Can you work these out from the model? Positions are in its coordinate system, mm. Coordinates: 2 decimals unless noted, no trailing zeros. Order: outer loops, then holes, each group sorted by start corner. A loop starts at its lowest first (then second) coordinate and runs counter-clockwise, first axis right, second up. Notation, with made-up numbers: (-35.5, -5.5) - (-15.5, -5.5) arc R30 cw to (-15.5, 16.5) - close; hole circle Ø6 at (-36.75, 38.5). An arc over 180 degrees is marked (long way). Return JSON: item names as keys, results as strings. Group by question number.
1) Imagine slicing it at B-B (y = 1.8). Give the number of separate pieces and of enclosed holes in the cut face, and give its area (3 significant figures).
2) For pin 1 Ø1.6 at (x, y) = (102, 1.5) entering from -Z; pin 2 Ø3 at (x, z) = (86.96, 38.69) entering from +Y; pin 3 Ø1.5 at (y, z) = (2.5, -19) entering from +X; pin 4 Ø0.6 at (x, y) = (102, 2) entering from +Z, each with a flat end and sliding along its axis, tell me the tip position at first contact or that it passes through.
3) If we mould it in two halves opening along Z, with no side actions, what happens to faces 1 (the face through (-83, 0, 41)), 2 (the face through (-172.517, 2.535, -37.813))? For each: pulls with the +Z half, pulls with the -Z half, needs draft (parallel to the pull), parting line crosses it, or undercut.
4) If I drill on line 1 along Z through (x, y) = (165.5, 4.15); line 2 along Z through (x, y) = (192, 3.5); line 3 along X through (y, z) = (3.85, 127), over which ranges is the centre line in solid material (lowest first)?
5) Imagine slicing it at A-A (z = -63.5). Write out the boundary of the cut face in (x, y), and give its area (3 significant figures).
6) Imagine slicing it at C-C (z = 20.5). Write out the boundary of the cut face in (x, y).
Autodesk Inventor part; units mm, degrees
ref_plane "Work Plane2" through (100.7136, 5, 38.6884) normal (0, 0, 1) x (1, 0, 0)
ref_plane "YZ Plane" through (0, 0, 0) normal (1, 0, 0) x (0, 1, 0)
ref_plane "XZ Plane" through (0, 0, 0) normal (0, 1, 0) x (-1, 0, 0)
sketch "Sketch1" plane through (0, 0, 0) normal (0, 1, 0) x (-1, 0, 0)
  line L0 (277.2864, 213.6884) -> (-214.7136, 213.6884)
  line L1 (-214.7136, -136.3116) -> (277.2864, -136.3116)
  line L2 (277.2864, -136.3116) -> (277.2864, 213.6884)
  line L3 (-214.7136, 159.6884) -> (-102.7136, 159.6884)
  line L4 (-102.7136, 159.6884) -> (-102.7136, -82.3116)
  line L5 (-102.7136, -82.3116) -> (-214.7136, -82.3116)
  line L6 (-214.7136, 213.6884) -> (-214.7136, 159.6884)
  line L7 (-214.7136, -82.3116) -> (-214.7136, -136.3116)
  point P0 (0, 0)
  dimension "d0" = 350
  dimension "d1" = 492
  dimension "d2" = 112
  dimension "d3" = 112
  dimension "d4" = 54
  dimension "d5" = 54
extrude "Extrusion1" add sketch "Sketch1" along normal blind 5
sketch "Sketch2" plane through (0, 5, 0) normal (0, 1, 0) x (1, 0, 0)
  line L0 (214.7136, 136.3116) -> (-277.2864, 136.3116)
  line L1 (-207.2864, 136.3116) -> (-137.2864, 136.3116)
  line L2 (-137.2864, 136.3116) -> (-137.2864, 134.3116)
  line L3 (-137.2864, 134.3116) -> (-207.2864, 134.3116)
  line L4 (-207.2864, 134.3116) -> (-207.2864, 136.3116)
  line L5 (-67.2864, 136.3116) -> (4.7136, 136.3116)
  line L6 (4.7136, 136.3116) -> (4.7136, 134.3116)
  line L7 (4.7136, 134.3116) -> (-67.2864, 134.3116)
  line L8 (-67.2864, 134.3116) -> (-67.2864, 136.3116)
  line L9 (74.7136, 136.3116) -> (144.7136, 136.3116)
  line L10 (144.7136, 136.3116) -> (144.7136, 134.3116)
  line L11 (144.7136, 134.3116) -> (74.7136, 134.3116)
  line L12 (74.7136, 134.3116) -> (74.7136, 136.3116)
  line L13 (-277.2864, -213.6884) -> (214.7136, -213.6884)
  line L14 (144.7136, -213.6884) -> (74.7136, -213.6884)
  line L15 (74.7136, -213.6884) -> (74.7136, -211.6884)
  line L16 (74.7136, -211.6884) -> (144.7136, -211.6884)
  line L17 (144.7136, -211.6884) -> (144.7136, -213.6884)
  line L18 (4.7136, -213.6884) -> (-67.2864, -213.6884)
  line L19 (-67.2864, -213.6884) -> (-67.2864, -211.6884)
  line L20 (-67.2864, -211.6884) -> (4.7136, -211.6884)
  line L21 (4.7136, -211.6884) -> (4.7136, -213.6884)
  line L22 (-137.2864, -213.6884) -> (-207.2864, -213.6884)
  line L23 (-207.2864, -213.6884) -> (-207.2864, -211.6884)
  line L24 (-207.2864, -211.6884) -> (-137.2864, -211.6884)
  line L25 (-137.2864, -211.6884) -> (-137.2864, -213.6884)
  line L26 (-277.2864, 136.3116) -> (-277.2864, -213.6884)
  line L27 (-277.2864, 86.3116) -> (-275.2864, 86.3116)
  line L28 (-275.2864, 86.3116) -> (-275.2864, 36.3116)
  line L29 (-275.2864, 36.3116) -> (-277.2864, 36.3116)
  line L30 (-277.2864, 36.3116) -> (-277.2864, 86.3116)
  line L31 (-277.2864, -13.6884) -> (-275.2864, -13.6884)
  line L32 (-275.2864, -13.6884) -> (-275.2864, -63.6884)
  line L33 (-275.2864, -63.6884) -> (-277.2864, -63.6884)
  line L34 (-277.2864, -63.6884) -> (-277.2864, -13.6884)
  line L35 (-277.2864, -113.6884) -> (-275.2864, -113.6884)
  line L36 (-275.2864, -113.6884) -> (-275.2864, -163.6884)
  line L37 (-275.2864, -163.6884) -> (-277.2864, -163.6884)
  line L38 (-277.2864, -163.6884) -> (-277.2864, -113.6884)
  line L39 (214.7136, 82.3116) -> (214.7136, 136.3116)
  line L40 (214.7136, 124.3116) -> (212.7136, 124.3116)
  line L41 (212.7136, 124.3116) -> (212.7136, 94.3116)
  line L42 (212.7136, 94.3116) -> (214.7136, 94.3116)
  line L43 (214.7136, 94.3116) -> (214.7136, 124.3116)
  line L44 (214.7136, -213.6884) -> (214.7136, -159.6884)
  line L45 (214.7136, -171.6884) -> (212.7136, -171.6884)
  line L46 (212.7136, -171.6884) -> (212.7136, -201.6884)
  line L47 (212.7136, -201.6884) -> (214.7136, -201.6884)
  line L48 (214.7136, -201.6884) -> (214.7136, -171.6884)
  line L49 (102.7136, 82.3116) -> (214.7136, 82.3116)
  line L50 (214.7136, -159.6884) -> (102.7136, -159.6884)
  line L51 (184.7136, 82.3116) -> (130.7136, 82.3116)
  line L52 (130.7136, 82.3116) -> (130.7136, 84.3116)
  line L53 (130.7136, 84.3116) -> (184.7136, 84.3116)
  line L54 (184.7136, 84.3116) -> (184.7136, 82.3116)
  line L55 (184.7136, -159.6884) -> (130.7136, -159.6884)
  line L56 (130.7136, -159.6884) -> (130.7136, -161.6884)
  line L57 (130.7136, -161.6884) -> (184.7136, -161.6884)
  line L58 (184.7136, -161.6884) -> (184.7136, -159.6884)
  line L59 (102.7136, -159.6884) -> (102.7136, 82.3116)
  line L60 (102.7136, 50.3116) -> (100.7136, 50.3116)
  line L61 (100.7136, 50.3116) -> (100.7136, 18.3116)
  line L62 (100.7136, 18.3116) -> (102.7136, 18.3116)
  line L63 (102.7136, 18.3116) -> (102.7136, 50.3116)
  line L64 (102.7136, -13.6884) -> (100.7136, -13.6884)
  line L65 (100.7136, -13.6884) -> (100.7136, -63.6884)
  line L66 (100.7136, -63.6884) -> (102.7136, -63.6884)
  line L67 (102.7136, -63.6884) -> (102.7136, -13.6884)
  line L68 (102.7136, -127.6884) -> (100.7136, -127.6884)
  line L69 (100.7136, -127.6884) -> (100.7136, -95.6884)
  line L70 (100.7136, -95.6884) -> (102.7136, -95.6884)
  line L71 (102.7136, -95.6884) -> (102.7136, -127.6884)
  point P0 (0, 0)
  point P1 (-207.2864, -213.6884)
  point P2 (130.7136, -159.6884)
  dimension "d8" = 2
  dimension "d9" = 2
  dimension "d10" = 2
  dimension "d11" = 2
  dimension "d12" = 50
  dimension "d13" = 50
  dimension "d14" = 50
  dimension "d15" = 50
  dimension "d16" = 50
  dimension "d17" = 50
  dimension "d18" = 12
  dimension "d19" = 12
  dimension "d20" = 12
  dimension "d21" = 12
  dimension "d22" = 70
  dimension "d23" = 70
  dimension "d24" = 72
  dimension "d25" = 70
  dimension "d26" = 70
  dimension "d27" = 70
  dimension "d28" = 2
  dimension "d29" = 2
  dimension "d30" = 30
  dimension "d32" = 2
  dimension "d33" = 2
  dimension "d34" = 2
  dimension "d35" = 32
  dimension "d36" = 32
  dimension "d37" = 32
  dimension "d39" = 32
  dimension "d40" = 32
  dimension "d41" = 32
  dimension "d42" = 50
  dimension "d45" = 72
  dimension "d46" = 70
  dimension "d47" = 28
  dimension "d48" = 28
  dimension "d49" = 54
  dimension "d50" = 54
  dimension "d51" = 30
extrude "Extrusion2" cut sketch "Sketch2" against normal blind 10 contours L10 L11 L12 L0 | L39 L42 L41 L40 | L6 L7 L8 L0 | L49 L52 L53 L54 | L2 L3 L4 L0 | L59 L62 L61 L60 | L27 L28 L29 L26 | L59 L66 L65 L64 | L31 L32 L33 L26 | L59 L68 L69 L70 | L35 L36 L37 L26 | L50 L58 L57 L56 | L23 L24 L25 L13 | L19 L20 L21 L13 | L44 L47 L46 L45 | L15 L16 L17 L13
sketch "Sketch3" plane through (0, 5, 0) normal (0, 1, 0) x (1, 0, 0)
  circle A0 centre (-177.2864, 36.3116) radius 5
  line L0 (-277.2864, 136.3116) -> (-277.2864, 86.3116)
  line L1 (-207.2864, 136.3116) -> (-277.2864, 136.3116)
  point P0 (0, 0)
  dimension "d52" = 100
  dimension "d53" = 100
  dimension "d54" = 10
extrude "Extrusion3" cut sketch "Sketch3" against normal blind 10
pattern_linear "Rectangular Pattern1" count 2 spacing 150 along (0, 0, 1) count 2 spacing 150 along (1, 0, 0) of "Extrusion3"
sketch "Sketch5" plane through (0, 5, 0) normal (0, 1, 0) x (1, 0, 0)
  circle A0 centre (87.1836, 43.3116) radius 1.9
  circle A1 centre (22.1836, 81.3116) radius 1.9
  circle A2 centre (-87.8164, 81.3116) radius 1.9
  line L0 (102.7136, 50.3116) -> (102.7136, 82.3116)
  line L1 (102.7136, -13.6884) -> (102.7136, 18.3116)
  line L2 (-67.2864, 136.3116) -> (-137.2864, 136.3116)
  line L3 (74.7136, 136.3116) -> (4.7136, 136.3116)
  point P0 (0, 0)
  dimension "d63" = 15.53
  dimension "d64" = 3.8
  dimension "d65" = 80.53
  dimension "d66" = 3.8
  dimension "d67" = 3.8
  dimension "d68" = 190.53
  dimension "d69" = 55
  dimension "d70" = 55
  dimension "d71" = 93
extrude "Extrusion4" cut sketch "Sketch5" against normal blind 10
sketch "Sketch6" plane through (0, 5, 0) normal (0, 1, 0) x (1, 0, 0)
  line L0 (100.7136, -63.6884) -> (100.7136, -13.6884)
  line L1 (100.7136, -38.6884) -> (-275.2864, -38.6884)
  line L2 (-275.2864, -63.6884) -> (-275.2864, -13.6884)
  point P0 (0, 0)
ref_plane "Work Plane2" through (100.7136, 5, 38.6884) normal (0, 0, 1) x (1, 0, 0)
mirror "Mirror1" about plane through (100.7136, 5, 38.6884) normal (0, 0, 1) of "Extrusion4"
sketch "Sketch8" plane through (0, 5, 0) normal (0, 1, 0) x (1, 0, 0)
  circle A0 centre (86.9636, -38.6884) radius 2.5
  circle A1 centre (30.4636, -38.6884) radius 2.5
  line L0 (130.7136, -159.6884) -> (102.7136, -159.6884)
  line L1 (102.7136, -95.6884) -> (102.7136, -63.6884)
  point P0 (0, 0)
  point P1 (116.7136, -159.6884)
  dimension "d78" = 5
  dimension "d79" = 121
  dimension "d80" = 121
  dimension "d81" = 15.75
  dimension "d82" = 56.5
  dimension "d83" = 5
extrude "Extrusion5" cut sketch "Sketch8" against normal blind 10
sketch "Sketch9" plane through (0, 5, 0) normal (0, 1, 0) x (1, 0, 0)
  circle A0 centre (59.7136, -97.6884) radius 8.5
  line L0 (4.7136, -213.6884) -> (74.7136, -213.6884)
  line L1 (102.7136, -95.6884) -> (102.7136, -63.6884)
  point P0 (0, 0)
  dimension "d86" = 17
  dimension "d87" = 116
  dimension "d88" = 43
extrude "Extrusion6" cut sketch "Sketch9" against normal blind 10
properties part number "top"
Calculated:
{
 "1": {"separate pieces": "1", "enclosed holes": "13", "area": "143,000 mm2"},
 "2": {"pin 1": "z = -134.31", "pin 2": "through", "pin 3": "x = 102.71", "pin 4": "z = 211.69"},
 "3": {"face 1": "needs draft", "face 2": "undercut"},
 "4": {"line 1": "-136.31 to -84.31, 161.69 to 213.69", "line 2": "-136.31 to -82.31, 159.69 to 213.69", "line 3": "-275.29 to 100.71"},
 "5": {"outline": "(-275.29, 0) - (102.71, 0) - (102.71, 5) - (-275.29, 5) - close", "area": "1,890 mm2"},
 "6": {"outline": "(-275.29, 0) - (100.71, 0) - (100.71, 5) - (-275.29, 5) - close"}
}
